from build123d import *

# Parameters (mm, degrees)
F3_DEPTH      = 25
F3_DEPTH_BACK = 25


with BuildPart() as f1:
    # F0 (on Front) → F1 (revolve)
    with BuildSketch(Plane.XZ):
        with BuildLine():
            Line((150, 5.75), (6.9236912121, 5.75))
            ThreePointArc((6.9236912121, 5.75), (-3.0566958543, 8.4650227675), (-9, 0))
            Line((-9, 0), (150, 0))
            Line((150, 0), (150, 5.75))
        make_face()
    revolve(axis=Axis((120.5487623811, 0, 0), (1, 0, 0)))

    # F2 (on Front) → F3 (cut, two sides)
    with BuildSketch(Plane.XZ) as f3_sk:
        Polygon((10, 9), (10, 10), (-10, 10), (-10, 5), (6, 5), align=None)
    extrude(amount=-F3_DEPTH, mode=Mode.SUBTRACT)
    extrude(f3_sk.sketch, amount=F3_DEPTH_BACK, mode=Mode.SUBTRACT)

    # F4 (on Front) → F5 (revolve, cut)
    with BuildSketch(Plane.XZ):
        Polygon((-5, -3.5), (0, -6.3867513459), (0, 5), (-5.7505553499, 5), (-5, 3.7), (-5.2, 3.5), (-6, 3.5), (-6, 0.5), (-5, 0.5), align=None)
    revolve(axis=Axis((0, 0, 6.4185173251), (0, 0, 1)), mode=Mode.SUBTRACT)


solid = f1.part
For this review, take the finished solid that the model builds, in its own axes (mm). A direction names the side the tool comes from. Coordinates: 2 decimals unless noted, no trailing zeros. Loops run counter-clockwise (first coordinate to the right, second up) from the corner with the lowest first, then second, coordinate; pieces in that order, holes last. Notation, with made-up numbers: (8.25, 24) - (26.25, 24) arc R27 ccw to (26.25, 56) - close; hole circle Ø7 at (51, -39). An arc over 180 degrees is marked (long way). Use a Markdown table: item, result. Add a question column.
Item 1: Mouldability with a two-part tool opening along Z and no side actions: class faces 5 (the face through (6, 0, 2)), 6 (the face through (1.08, 4.88, -1.53)), 7 (the face through (0.634, 0.486, -5.926)) as pulls with the +Z half, pulls with the -Z half, needs draft (parallel to the pull), parting line crosses it, or undercut.
Item 2: Insertion check: pin 1 Ø1.5 at (x, z) = (128.5, 1.5) entering from +Y; pin 2 Ø2 at (x, z) = (79, -5.5) entering from +Y; pin 3 Ø9 at (x, y) = (0, 0) entering from +Z. Each pin has a flat end and moves straight along its axis. Give the tip position at first contact, or say it passes through.
Item 3: For line 1 (Y direction, x = 0, z = -0.65); line 2 (Y direction, x = -2, z = -0.75); line 3 (X direction, y = 0, z = -2.6), list the stretches that pass through material, from the lowest coordinate up.
Item 4: We need section A-A (x = 134.5). Give the boundary of the cut face in (y, z).
Item 5: Tool access review of faces 1 (the face through (150, 0, 0)), 2 (the face through (77.46, -5.7, -0.75)), 3 (the face through (-2, -5, 3.5)), 4 (the face through (-6, 0, 5)): name each direction out of +Z, -Z, +X, -X, +Y, -Y from which nothing blocks a thin tool from reaching the whole face with its end or side.
Results list:
| question | item | result |
|---|---|---|
| 1 | face 5 | undercut |
| 1 | face 6 | needs draft |
| 1 | face 7 | pulls with the +Z half |
| 2 | pin 1 | stops at y = 5.7 |
| 2 | pin 2 | stops at y = 3.58 |
| 2 | pin 3 | stops at z = -3.79 |
| 3 | line 1 | y = -8.98 to -5, 5 to 8.98 |
| 3 | line 2 | y = -8.74 to -4.58, 4.58 to 8.74 |
| 3 | line 3 | x = -8.62 to -5, 5 to 150 |
| 4 | outline | circle Ø11.5 at (0, 0) |
| 5 | face 1 | +Z, -Z, +X, +Y, -Y |
| 5 | face 2 | +X |
| 5 | face 3 | none |
| 5 | face 4 | +Z, -X, +Y, -Y |
